Can you work these out from the model? Positions are in its coordinate system, mm. A direction names the side the tool comes from. Round coordinates to 2 decimals unless told otherwise and drop trailing zeros. Loops run counter-clockwise (first coordinate to the right, second up) from the corner with the lowest first, then second, coordinate; pieces in that order, holes last.
(1) I want a section at A-A on y = 7.5. Write out the boundary of the cut face in (x, z), plus the area to 3 significant figures.
(2) If I drill on line 1 along Z through (x, y) = (0, 22); line 2 along X through (y, z) = (3.5, 12.5); line 3 along Z through (x, y) = (0, 17), over which ranges is the centre line in solid material (lowest first)?
(3) Thinking about a two-plate mould opening in Y: for faces 1 (the face through (-9.641, 19.203, 7.395)), 2 (the face through (14.68, -14.65, 7.4)), 3 (the face through (3, 15.25, 7)), 4 (the face through (18, 3, 7)), which applies, released by +Y, released by -Y, zero draft, split by the parting line, or undercut?
(4) I want a section at D-D on y = 21. Write out the boundary of the cut face in (x, z), plus the area to 3 significant figures.
(5) I want a section at B-B on x = 0. Write out the boundary of the cut face in (y, z), plus the area to 3 significant figures.
(6) I want a section at C-C on x = 11. Write out the boundary of the cut face in (y, z), plus the area to 3 significant figures.
(7) Will these pins go through, and if not, where does the flat tip stop? pin 1 Ø2 at (y, z) = (23, 9) entering from +X; pin 2 Ø6 at (y, z) = (-9.5, 1.5) entering from -X; pin 3 Ø5 at (y, z) = (14, 9.5) entering from -X.
(8) Which directions (+Z, -Z, +X, -X, +Y, -Y) give clear straight access to the entire face, cutting with the end or side of a thin tool? Please do faces 5 (the face through (20, -29.3, 8)), 6 (the face through (-14, 18, 7)), 7 (the face through (14, 18, 7)).
from build123d import *

# Parameters (mm, degrees)
F1_DEPTH       = 15
F2_T1_DEPTH    = 24.3030738828
F4_R           = 5.5
F5_DEPTH       = 6
F6_R           = 1
F7_R           = 2.1
F8_DEPTH       = 3.75
F9_R           = 5.5
F10_DEPTH      = 10
F10_DEPTH_BACK = 25
F11_R          = 2.1
F12_DEPTH      = 14.75
F3_R           = 2.8
F13_DEPTH      = 6.5
F14_R          = 4.4
F15_DEPTH      = 0.7


# Not quite as in the source:
# - a fillet or chamfer that OpenCascade refuses, or shapes differently, is made with other operations: its cross-section is extruded or revolved along the edge and cut away or added


with BuildPart() as f1:
    # F0 (on Top) → F1 (new body)
    with BuildSketch(Plane.XY):
        with BuildLine():
            ThreePointArc((18, 16), (17.4142135624, 17.4142135624), (16, 18))
            Line((16, 18), (12.5, 18))
            ThreePointArc((12.5, 18), (9.6715728753, 19.1715728753), (8.5, 22))
            Line((8.5, 22), (8.5, 25))
            Line((8.5, 25), (-8.5, 25))
            Line((-8.5, 25), (-8.5, 22))
            ThreePointArc((-8.5, 22), (-9.6715728753, 19.1715728753), (-12.5, 18))
            Line((-12.5, 18), (-16, 18))
            ThreePointArc((-16, 18), (-17.4142135624, 17.4142135624), (-18, 16))
            Line((-18, 16), (-18, -10))
            ThreePointArc((-18, -10), (-20.3431457505, -15.6568542495), (-26, -18))
            Line((-26, -18), (-26, -30))
            Line((-26, -30), (26, -30))
            Line((26, -30), (26, -18))
            ThreePointArc((26, -18), (20.3431457505, -15.6568542495), (18, -10))
            Line((18, -10), (18, 16))
        make_face()
        with BuildLine():
            Line((-13.25, 15.25), (13.25, 15.25))
            ThreePointArc((13.25, 15.25), (14.6642135624, 14.6642135624), (15.25, 13.25))
            Line((15.25, 13.25), (15.25, -13.25))
            ThreePointArc((15.25, -13.25), (14.6642135624, -14.6642135624), (13.25, -15.25))
            Line((13.25, -15.25), (-13.25, -15.25))
            ThreePointArc((-13.25, -15.25), (-14.6642135624, -14.6642135624), (-15.25, -13.25))
            Line((-15.25, -13.25), (-15.25, 13.25))
            ThreePointArc((-15.25, 13.25), (-14.6642135624, 14.6642135624), (-13.25, 15.25))
        make_face(mode=Mode.SUBTRACT)
    extrude(amount=F1_DEPTH)

    # F2: chamfer of 2 on 2 edges, made by hand

    # F2_s2 → F2_t1 (cut)
    with BuildSketch(Plane.XY.offset(-4.6515369414)):
        with BuildLine():
            Line((-24.4, -17.8383671769), (-26, -19.7979589711))
            Line((-26, -19.7979589711), (-26, -18))
            ThreePointArc((-26, -18), (-25.1675484588, -17.9565711479), (-24.4, -17.8383671769))
        make_face()
        with BuildLine():
            Line((26, -19.7979589711), (24.4, -17.8383671769))
            ThreePointArc((24.4, -17.8383671769), (25.1675484588, -17.9565711479), (26, -18))
            Line((26, -18), (26, -19.7979589711))
        make_face()
    extrude(amount=F2_T1_DEPTH, mode=Mode.SUBTRACT)

    # F4 (on face) → F5 (cut)
    with BuildSketch(Plane(origin=(0, 25, 0), x_dir=(-1, 0, 0), z_dir=(0, 1, 0))):
        with Locations((0, 7.5)):
            Circle(F4_R)
    extrude(amount=-F5_DEPTH, mode=Mode.SUBTRACT)

    # F6
    f6_edges = [f1.edges().sort_by_distance(p)[0] for p in [
        (0, 25, 0),
        (-8.5, 25, 7.5),
        (0, 25, 15),
        (8.5, 25, 7.5),
    ]]
    fillet(f6_edges, radius=F6_R)

    # F7 (on face) → F8 (cut, through all)
    with BuildSketch(Plane(origin=(0, 19, 0), x_dir=(-1, 0, 0), z_dir=(0, 1, 0))):
        with Locations((0, 7.5)):
            Circle(F7_R)
    extrude(amount=-F8_DEPTH, mode=Mode.SUBTRACT)

    # F9 (on face) → F10 (cut, two sides)
    with BuildSketch(Plane.XZ.offset(30)) as f10_sk:
        with Locations((0, 7.5)):
            Circle(F9_R)
    extrude(amount=-F10_DEPTH, mode=Mode.SUBTRACT)
    extrude(f10_sk.sketch, amount=F10_DEPTH_BACK, mode=Mode.SUBTRACT)

    # F11 (on face) → F12 (cut, through all)
    with BuildSketch(Plane.XZ.offset(30)):
        with Locations((0, 7.5)):
            Circle(F11_R)
    extrude(amount=-F12_DEPTH, mode=Mode.SUBTRACT)

    # F3 (on face) → F13 (cut)
    with BuildSketch(Plane.XZ.offset(30)):
        with Locations((-17, 7.5)):
            Circle(F3_R)
        with Locations((17, 7.5)):
            Circle(F3_R)
    extrude(amount=-F13_DEPTH, mode=Mode.SUBTRACT)

    # F14 (on face) → F15 (cut)
    with BuildSketch(Plane.XZ.offset(30)):
        with Locations((17, 7.5)):
            Circle(F14_R)
        with Locations((-17, 7.5)):
            Circle(F14_R)
    extrude(amount=-F15_DEPTH, mode=Mode.SUBTRACT)


solid = f1.part
Filled sheet:
1. outline: (-18, 0) - (-15.25, 0) - (-15.25, 15) - (-18, 15) - close; (15.25, 0) - (18, 0) - (18, 15) - (15.25, 15) - close
1. area: 82.5 mm2
2. line 1: z = 0 to 2, 13 to 15
2. line 2: x = -18 to -15.25, 15.25 to 18
2. line 3: z = 0 to 5.4, 9.6 to 15
3. face 1: released by +Y
3. face 2: undercut
3. face 3: undercut
3. face 4: zero draft
4. outline: (-8.63, 0) - (8.63, 0) - (8.63, 15) - (-8.63, 15) - close; hole circle Ø11 at (0, 7.5)
4. area: 164 mm2
5. outline: (-30, 0) - (-15.25, 0) - (-15.25, 5.4) - (-20, 5.4) - (-20, 2) - (-30, 2) - close; (-30, 13) - (-20, 13) - (-20, 9.6) - (-15.25, 9.6) - (-15.25, 15) - (-30, 15) - close; (15.25, 0) - (24, 0) arc R1 ccw to (25, 1) - (25, 2) - (19, 2) - (19, 5.4) - (15.25, 5.4) - close; (15.25, 9.6) - (19, 9.6) - (19, 13) - (25, 13) - (25, 14) arc R1 ccw to (24, 15) - (15.25, 15) - close
5. area: 155 mm2
6. outline: (-30, 0) - (-15.25, 0) - (-15.25, 15) - (-30, 15) - close; (15.25, 0) - (18.29, 0) - (18.29, 15) - (15.25, 15) - close
6. area: 267 mm2
7. pin 1: stops at x = 8.5
7. pin 2: stops at x = -18.4
7. pin 3: stops at x = -18
8. face 5: -Y
8. face 6: +Z, -Z, -X, +Y
8. face 7: +Z, -Z, +X, +Y
